Study the drawing (mm; zero at the part's minimum x, y, z) and answer. Round coordinates to 2 decimals unless told otherwise and drop trailing zeros. Write each loop counter-clockwise with the first axis right and the second up, starting at its lowest first coordinate (ties: lowest second). Pieces come first, ordered by that corner, then holes.
(1) A cutting plane is placed at C-C, the plane z = 3.75. Give the vertices of the cut face in (x, y), and give its area (3 significant figures).
(2) A cutting plane is placed at D-D, the plane x = 4.35. Give the vertices of the cut face in (y, z), and give its area (3 significant figures).
(3) Find the intervals of material crossed by probe 1 along X at (y, z) = (2.6, 6); probe 2 along X at (y, z) = (2.1, 3.25), in increasing order.
(4) A cutting plane is placed at A-A, the plane y = 2.5. Give the vertices of the cut face in (x, z), and give its area (3 significant figures).
(5) Each of these flat-tipped pins is pushed along its axis until it touches: pin 1 Ø2 at (x, y) = (2, 0.5) entering from -Z; pin 2 Ø1.5 at (y, z) = (0.5, 5.5) entering from +X. Where does it stop, or does it pass through?
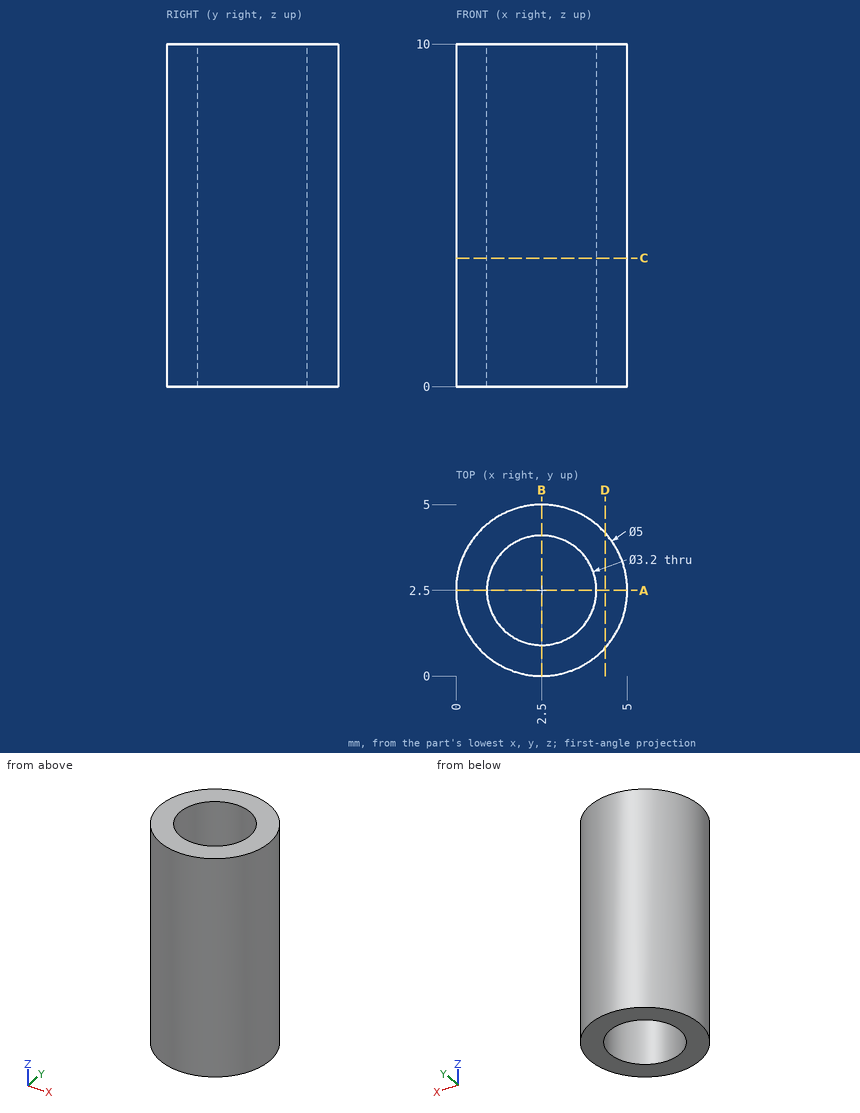
Solutions:
1. outline: circle Ø5 at (2.5, 2.5); hole circle Ø3.2 at (2.5, 2.5)
1. area: 11.6 mm2
2. outline: (0.82, 0) - (4.18, 0) - (4.18, 10) - (0.82, 10) - close
2. area: 33.6 mm2
3. probe 1: x = 0 to 0.9, 4.1 to 5
3. probe 2: x = 0.03 to 0.95, 4.05 to 4.97
4. outline: (0, 0) - (0.9, 0) - (0.9, 10) - (0, 10) - close; (4.1, 0) - (5, 0) - (5, 10) - (4.1, 10) - close
4. area: 18.0 mm2
5. pin 1: stops at z = 0
5. pin 2: stops at x = 4.67
